Design review of the part built by this model. Coordinates are the model's own, in mm. Round coordinates to 2 decimals unless told otherwise and drop trailing zeros. Loops run counter-clockwise (first coordinate to the right, second up) from the corner with the lowest first, then second, coordinate; pieces in that order, holes last. Notation, with made-up numbers: (0.25, -32) - (54.25, -32) arc R23 cw to (54.25, -12) - close; hole circle Ø11 at (36.5, -14). An arc over 180 degrees is marked (long way). Return JSON: item names as keys, results as strings. Group by question number.
(1) We need section C-C, the plane x = -26.15. Write out the cut boundary in (y, z).
(2) Wall thickness on L1, parallel to X at y = 5.9, z = 6; L2, parallel to Y at x = -24.35, z = 11; L3, parallel to X at y = 5.6, z = 16: over which ranges is each line inside the solid? List them lowest first. Write a range as [from, to].
(3) We need section B-B, the plane z = -3. Write out the cut boundary in (x, y), and give its area (3 significant figures).
(4) Clearance check with flat-ended pins moving along their axes: pin 1 (1.5 mm diameter, centred on x = -24, y = 5.5, fed in from +Z); pin 2 (1 mm diameter, centred on x = -24, z = 10, fed in from +Y). State where each tip first meets the part, or that it passes through.
(5) We need section A-A, the plane y = 5. Write out the cut boundary in (x, z), and give its area (3 significant figures).
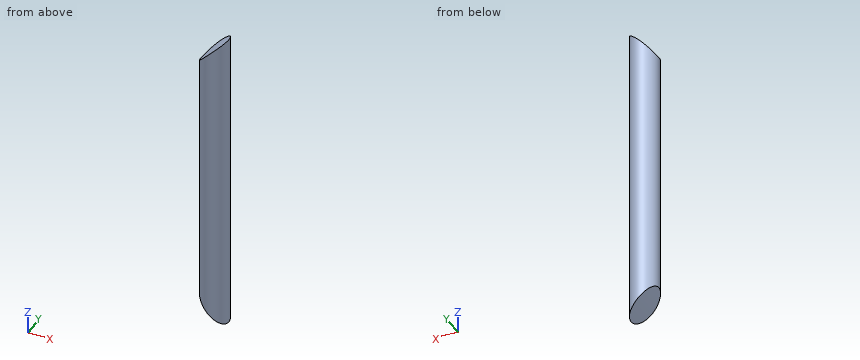
from build123d import *

# Parameters (mm, degrees)
BOSS_EXTRUDE1_DEPTH      = 40
BOSS_EXTRUDE1_DEPTH_BACK = 40
SKETCH3_R                = 2.4
CUT_EXTRUDE1_START       = 2.6
SKETCH1_R                = 50
SKETCH1_R_2              = 35
CUT_EXTRUDE1_DEPTH       = 4.8
SCALE1_SCALE             = 0.8


with BuildPart() as part:
    # Sketch3 → Boss-Extrude1 (new, two sides: drawn at the far end of the back side and taken through both)
    with BuildSketch(Plane.XY.offset(-BOSS_EXTRUDE1_DEPTH_BACK)):
        with Locations((-25, 5)):
            Circle(SKETCH3_R)
    extrude(amount=BOSS_EXTRUDE1_DEPTH + BOSS_EXTRUDE1_DEPTH_BACK)

    # Sketch1 → Cut-Extrude1 (cut)
    with BuildSketch(Plane(origin=(0, 0, 0), x_dir=(1, 0, 0), z_dir=(0, 1, 0)).offset(CUT_EXTRUDE1_START)):
        Circle(SKETCH1_R)
        Circle(SKETCH1_R_2, mode=Mode.SUBTRACT)
    extrude(amount=CUT_EXTRUDE1_DEPTH, mode=Mode.SUBTRACT)


with BuildPart() as part_1:
    # Scale1: scaled about (-24.939549166, 4.999999342, -0.000153755)
    add(part.part.scale(SCALE1_SCALE).moved(Location((-4.987909833, 0.999999868, -3.0751e-05))))


solid = part_1.part
Solutions:
{
 "1": {"outline": "(3.47, -18.33) - (6.53, -18.33) - (6.53, 18.33) - (3.47, 18.33) - close"},
 "2": {"L1": "[-26.68, -23.29]", "L2": "[3.19, 6.81]", "L3": "[-26.81, -23.16]"},
 "3": {"outline": "circle Ø3.84 at (-24.99, 5)", "area": "11.6 mm^2"},
 "4": {"pin 1": "z = 21.22", "pin 2": "y = 6.86"},
 "5": {"outline": "(-26.91, -17.42) arc R28 ccw to (-23.07, -21.38) - (-23.07, 21.38) arc R28 ccw to (-26.91, 17.42) - close", "area": "150 mm^2"}
}
